Check sheet for the modelled part. Datum: model origin and axes. Units: mm. Face numbers are marked on the shaded views. A direction names the side the tool comes from. Round coordinates to 2 decimals unless told otherwise and drop trailing zeros. Write each loop counter-clockwise with the first axis right and the second up, starting at its lowest first coordinate (ties: lowest second). Pieces come first, ordered by that corner, then holes.
Item 1: Cross-section at A-A on y = -27.5. Enter the section's corners in (x, z), plus the area to 3 significant figures.
Item 2: Cross-section at D-D on x = -65. Enter the section's corners in (y, z).
Item 3: Go/stop test with flat-tipped pins: pin 1 Ø1.5 at (x, z) = (14, -62) entering from -Y; pin 2 Ø11 at (x, z) = (64, -14) entering from -Y; pin 3 Ø3 at (x, z) = (-64, -13) entering from -Y; pin 4 Ø2 at (x, z) = (12.5, -54) entering from +Y. Record where each tip stops, or that it passes through.
Item 4: Cross-section at B-B on z = -61. Enter the section's corners in (x, y).
Item 5: Tool access check on the marked faces 4, 5 and 6. Record the directions out of +Z, -Z, +X, -X, +Y, -Y that give a thin tool (end or side, any length) a straight path to the whole face; none if there is none.
Item 6: Release check for a two-part mould opening along Z. For the marked faces 1, 2 and 3 record: +Z half, -Z half, draft (parallel to the pull), parting line (faces both ways), or undercut.
Item 7: Cross-section at C-C on x = 50.5. Enter the section's corners in (y, z).
Item 8: Material ranges on line 1 (X direction, y = -32, z = -111); line 2 (Y direction, x = -64, z = -56); line 3 (Y direction, x = -26, z = -44), recorded low to high.
from build123d import *

# Parameters (mm, degrees)
SKETCH1_W           = 160
SKETCH1_H           = 80
BOSS_EXTRUDE1_DEPTH = 126
SKETCH2_W           = 90
SKETCH2_H           = 60
CUT_EXTRUDE1_DEPTH  = 126
SKETCH3_R           = 5
CUT_EXTRUDE2_DEPTH  = 40
SHELL1_DEPTH        = 40
SHELL1_START        = -30
SHELL1_2_DEPTH      = 30
SHELL1_START_2      = 10
SHELL1_3_DEPTH      = 30
SKETCH4_W           = 110
SKETCH4_H           = 106
CUT_EXTRUDE3_DEPTH  = 10
SKETCH5_W           = 15
SKETCH5_H           = 73.639320226
CUT_EXTRUDE4_DEPTH  = 40


# Read off the part's stored shape, not the designer's step: Shell1
with BuildPart() as part:
    # Sketch1 → Boss-Extrude1 (new body)
    with BuildSketch(Plane.XY):
        Rectangle(SKETCH1_W, SKETCH1_H)
    extrude(amount=-BOSS_EXTRUDE1_DEPTH)

    # Sketch2 → Cut-Extrude1 (cut)
    with BuildSketch(Plane.XY):
        with Locations((0, -40)):
            Rectangle(SKETCH2_W, SKETCH2_H)
    extrude(amount=-CUT_EXTRUDE1_DEPTH, mode=Mode.SUBTRACT)

    # Sketch3 → Cut-Extrude2 (cut)
    with BuildSketch(Plane.XZ.offset(40)):
        with Locations(Location((-65, -15, 0), (0, 0, 270))):
            Circle(SKETCH3_R)
        with Locations(Location((65, -15, 0), (0, 0, 90))):
            Circle(SKETCH3_R)
        with Locations(Location((65, -111, 0), (0, 0, 270))):
            Circle(SKETCH3_R)
        with Locations(Location((-65, -111, 0), (0, 0, 90))):
            Circle(SKETCH3_R)
    extrude(amount=-CUT_EXTRUDE2_DEPTH, mode=Mode.SUBTRACT)

    # Shell1 outline → Shell1 (cut)
    with BuildSketch(Plane(origin=(0, 0, 0), x_dir=(1, 0, 0), z_dir=(0, 1, 0))):
        with BuildLine():
            Line((70, 29.142135624), (70, 96.857864376))
            ThreePointArc((70, 96.857864376), (54.393398282, 100.393398282), (50.857864376, 116))
            Line((50.857864376, 116), (-50.857864376, 116))
            ThreePointArc((-50.857864376, 116), (-54.393398282, 100.393398282), (-70, 96.857864376))
            Line((-70, 96.857864376), (-70, 29.142135624))
            ThreePointArc((-70, 29.142135624), (-54.393398282, 25.606601718), (-50.857864376, 10))
            Line((-50.857864376, 10), (50.857864376, 10))
            ThreePointArc((50.857864376, 10), (54.393398282, 25.606601718), (70, 29.142135624))
        make_face()
    extrude(amount=SHELL1_DEPTH, mode=Mode.SUBTRACT)

    # Shell1 2 outline → Shell1 2 (cut)
    with BuildSketch(Plane(origin=(0, 0, 0), x_dir=(1, 0, 0), z_dir=(0, 1, 0)).offset(SHELL1_START)):
        with BuildLine():
            ThreePointArc((55, 26.180339887), (62.094305849, 29.715873794), (70, 29.142135624))
            Line((70, 29.142135624), (70, 96.857864376))
            ThreePointArc((70, 96.857864376), (62.094305849, 96.284126206), (55, 99.819660113))
            Line((55, 99.819660113), (55, 26.180339887))
        make_face()
        with BuildLine():
            ThreePointArc((-70, 29.142135624), (-62.094305849, 29.715873794), (-55, 26.180339887))
            Line((-55, 26.180339887), (-55, 99.819660113))
            ThreePointArc((-55, 99.819660113), (-62.094305849, 96.284126206), (-70, 96.857864376))
            Line((-70, 96.857864376), (-70, 29.142135624))
        make_face()
    extrude(amount=SHELL1_2_DEPTH, mode=Mode.SUBTRACT)

    # Shell1 3 outline → Shell1 3 (cut)
    with BuildSketch(Plane(origin=(0, 0, 0), x_dir=(1, 0, 0), z_dir=(0, 1, 0)).offset(SHELL1_START_2)):
        with BuildLine():
            Line((50.857864376, 10), (70, 10))
            Line((70, 10), (70, 29.142135624))
            ThreePointArc((70, 29.142135624), (54.393398282, 25.606601718), (50.857864376, 10))
        make_face()
        with BuildLine():
            ThreePointArc((50.857864376, 116), (54.393398282, 100.393398282), (70, 96.857864376))
            Line((70, 96.857864376), (70, 116))
            Line((70, 116), (50.857864376, 116))
        make_face()
        with BuildLine():
            Line((-70, 10), (-50.857864376, 10))
            ThreePointArc((-50.857864376, 10), (-54.393398282, 25.606601718), (-70, 29.142135624))
            Line((-70, 29.142135624), (-70, 10))
        make_face()
        with BuildLine():
            ThreePointArc((-70, 96.857864376), (-54.393398282, 100.393398282), (-50.857864376, 116))
            Line((-50.857864376, 116), (-70, 116))
            Line((-70, 116), (-70, 96.857864376))
        make_face()
    extrude(amount=SHELL1_3_DEPTH, mode=Mode.SUBTRACT)

    # Sketch4 → Cut-Extrude3 (cut)
    with BuildSketch(Plane(origin=(0, 0, 0), x_dir=(1, 0, 0), z_dir=(0, 1, 0))):
        with Locations((0, 63)):
            Rectangle(SKETCH4_W, SKETCH4_H)
    extrude(amount=CUT_EXTRUDE3_DEPTH, mode=Mode.SUBTRACT)

    # Sketch5 → Cut-Extrude4 (cut)
    with BuildSketch(Plane(origin=(0, -30, 0), x_dir=(1, 0, 0), z_dir=(0, 1, 0))):
        with Locations((-62.5, 63)):
            Rectangle(SKETCH5_W, SKETCH5_H)
    cut_extrude4 = extrude(amount=CUT_EXTRUDE4_DEPTH, mode=Mode.SUBTRACT)

    # Mirror1: Cut-Extrude4 across plane
    add(cut_extrude4.mirror(Plane(origin=(0, 0, 0), x_dir=(0, 0, 1), z_dir=(1, 0, 0))), mode=Mode.SUBTRACT)


solid = part.part
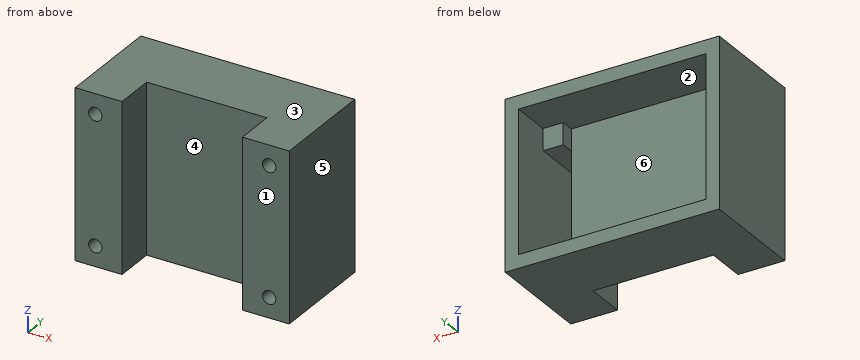
Response values:
1. outline: (-80, -126) - (-45, -126) - (-45, 0) - (-80, 0) - close; (45, -126) - (80, -126) - (80, 0) - (45, 0) - close; hole circle Ø10 at (-65, -111); hole (-70, -99.82) - (-55, -99.82) - (-55, -26.18) - (-70, -26.18) - close; hole circle Ø10 at (-65, -15); hole (55, -99.82) - (70, -99.82) - (70, -26.18) - (55, -26.18) - close; hole circle Ø10 at (65, -111); hole circle Ø10 at (65, -15)
1. area: 6,300 mm2
2. outline: (-40, -126) - (40, -126) - (40, -116) - (10, -116) - (10, -99.82) - (-30, -99.82) - (-30, -26.18) - (10, -26.18) - (10, -10) - (40, -10) - (40, 0) - (-40, 0) - (-40, -10) - (0, -10) - (0, -20) - (-40, -20) - (-40, -106) - (0, -106) - (0, -116) - (-40, -116) - close
3. pin 1: stops at y = -10
3. pin 2: stops at y = -40
3. pin 3: stops at y = 0
3. pin 4: stops at y = 0
4. outline: (-80, -40) - (-45, -40) - (-45, -10) - (45, -10) - (45, -40) - (80, -40) - (80, 40) - (70, 40) - (70, -30) - (55, -30) - (55, 0) - (-55, 0) - (-55, -30) - (-70, -30) - (-70, 40) - (-80, 40) - close
5. face 4: +Z, -Z, -Y
5. face 5: +Z, -Z, +X, +Y, -Y
5. face 6: +Y
6. face 1: draft
6. face 2: undercut
6. face 3: +Z half
7. outline: (-40, -126) - (40, -126) - (40, -116) - (0, -116) - (0, -10) - (40, -10) - (40, 0) - (-40, 0) - close
8. line 1: x = -80 to -70, -60 to -45, 45 to 60, 70 to 80
8. line 2: y = -40 to -30
8. line 3: y = -10 to 0
